from build123d import *

# Parameters (mm, degrees)
SKETCH1_R           = 1.5
BOSS_EXTRUDE1_DEPTH = 4
FILLET1_R           = 3


with BuildPart() as part:
    # Sketch1 → Boss-Extrude1 (new body)
    with BuildSketch(Plane.XY):
        with BuildLine():
            Line((0, 0), (48, 0))
            Line((48, 0), (48, 6))
            Line((48, 6), (39, 6))
            Line((39, 6), (39, 12))
            ThreePointArc((39, 12), (35.661193516, 15.944974415), (31.218588433, 13.304195753))
            ThreePointArc((31.218588433, 13.304195753), (29.055123964, 10.641481887), (25.684793917, 10))
            Line((25.684793917, 10), (-7.786766468, 15.474289455))
            ThreePointArc((-7.786766468, 15.474289455), (-10.94056647, 13.882322422), (-10.392304845, 10.392304845))
            Line((-10.392304845, 10.392304845), (0, 0))
        make_face()
        with Locations((35, 12)):
            Circle(SKETCH1_R, mode=Mode.SUBTRACT)
        with Locations((-8.270984502, 12.513625189)):
            Circle(SKETCH1_R, mode=Mode.SUBTRACT)
        with Locations((35, 3)):
            Circle(SKETCH1_R, mode=Mode.SUBTRACT)
        with Locations((45, 3)):
            Circle(SKETCH1_R, mode=Mode.SUBTRACT)
    extrude(amount=BOSS_EXTRUDE1_DEPTH)

    # Fillet1
    fillet1_edges = [part.edges().sort_by_distance(p)[0] for p in [
        (48, 0, 2),
        (48, 6, 2),
        (39, 6, 2),
        (0, 0, 2),
    ]]
    fillet(fillet1_edges, radius=FILLET1_R - 0.0001)  # a hair under: the kernel refuses the full size


solid = part.part
CAD build for the part. Positions are in the model's coordinates, mm. A direction names the side the tool comes from. Round coordinates to 2 decimals unless told otherwise and drop trailing zeros. Loops run counter-clockwise (first coordinate to the right, second up) from the corner with the lowest first, then second, coordinate; pieces in that order, holes last.
(1) Which spindle directions (+Z, -Z, +X, -X, +Y, -Y) get a long thin tool onto all of the face, cutting with end or side? Do faces 1 (the cylindrical face through (47.1, 0.86, 2.03)), 2 (the flat face through (44, 6, 2)), 3 (the flat face through (9.18, 12.7, 1.97)). Say none if no direction does.
(2) Cut at A-A (x = 35). Give the cut face in (y, z), plus the area to 3 significant figures.
(3) Drop flat-ended pins along their axis: pin 1 (4 mm diameter, centred on x = 35, y = 12, fed in from -Z); pin 2 (2.5 mm diameter, centred on x = 35, y = 3, fed in from +Z); pin 3 (1 mm diameter, centred on y = 13, z = 0.5, fed in from +X). Give the stop position or say it passes through.
(4) Cut at C-C (z = 0.65). State how many separate pieces and enclosed holes the cut face has, plus the area to 3 significant figures.
(5) Two-plate mould, pull along Y, no slides. Class faces 4 (the cylindrical face through (33.8, 11.1, 2)), 5 (the cylindrical face through (0.11, 0.22, 2.03)), 6 (the flat face through (39, 10, 2)), 7 (the cylindrical face through (33.8, 2.1, 2)): +Y half, -Y half, draft (parallel to the pull), parting line (faces both ways), or undercut.
(6) Wall check: line 1 along Y through (x, z) = (35, 2.65); line 2 along Y through (x, z) = (45, 1.65); line 3 along X through (y, z) = (2.5, 2.3). Give the ranges that are in metal, low to high.
(7) Cut at B-B (y = 3.75). Give the cut face in (x, z), plus the area to 3 significant figures.
(8) Cut at D-D (x = -4). Give the cut face in (y, z), plus the area to 3 significant figures.
Findings below:
1. face 1: +Z, -Z, +X, -Y
1. face 2: +Z, -Z, +X, +Y
1. face 3: +Z, -Z, +Y
2. outline: (0, 0) - (1.5, 0) - (1.5, 4) - (0, 4) - close; (4.5, 0) - (10.5, 0) - (10.5, 4) - (4.5, 4) - close; (13.5, 0) - (16, 0) - (16, 4) - (13.5, 4) - close
2. area: 40.0 mm2
3. pin 1: stops at z = 0
3. pin 2: passes through
3. pin 3: stops at x = 38.97
4. separate pieces: 1
4. enclosed holes: 4
4. area: 616 mm2
5. face 4: undercut
5. face 5: -Y half
5. face 6: draft
5. face 7: undercut
6. line 1: y = 0 to 1.5, 4.5 to 10.5, 13.5 to 16
6. line 2: y = 0 to 1.5, 4.5 to 6
6. line 3: x = -2.5 to 33.59, 36.41 to 43.59, 46.41 to 47.96
7. outline: (-3.75, 0) - (33.7, 0) - (33.7, 4) - (-3.75, 4) - close; (36.3, 0) - (43.7, 0) - (43.7, 4) - (36.3, 4) - close; (46.3, 0) - (47.9, 0) - (47.9, 4) - (46.3, 4) - close
7. area: 186 mm2
8. outline: (4, 0) - (14.85, 0) - (14.85, 4) - (4, 4) - close
8. area: 43.4 mm2
